Drawing for the job (mm, zero at the part's lowest x, y, z). Give positions to 0.01 mm unless a question says otherwise; leave off trailing zeros. Order: outer loops, then holes, each group sorted by start corner. A loop starts at its lowest first (then second) coordinate and runs counter-clockwise, first axis right, second up. Notation, with made-up numbers: (23, 77.5) -> (54, 77.5) arc R15 ccw to (54, 99.5) -> close; hole circle Ø8 at (36, -36). An arc over 180 degrees is marked (long way). One line per item, written item: value. Start each with the question number.
(1) Two-plate mould, pull along X, no slides. Class the marked faces 1, 2 and 3: +X half, -X half, draft (parallel to the pull), parting line (faces both ways), or undercut.
(2) Probe line 1 (Z direction, x = 21.5, y = 1.85); line 2 (Z direction, x = 17.5, y = 0.5); line 3 (Y direction, x = 17.5, z = 1.9). List the from-to ranges inside material, lowest first.
(3) Saw through at A-A on y = 2. Give the cut face in (x, z).
(4) Saw through at B-B on x = 16.75. Give the cut face in (y, z), plus the area to 3 significant figures.
(5) Pin check, flat tips, straight feed: pin 1 (0.6 mm diameter, centred on y = 1.5, z = 4, fed in from -X); pin 2 (1.5 mm diameter, centred on x = 14, z = 3, fed in from -Y); pin 3 (0.6 mm diameter, centred on y = 1.5, z = 3.5, fed in from +X); pin 4 (1 mm diameter, centred on x = 14, y = 1, fed in from -Z). Stop position of each tip, or through.
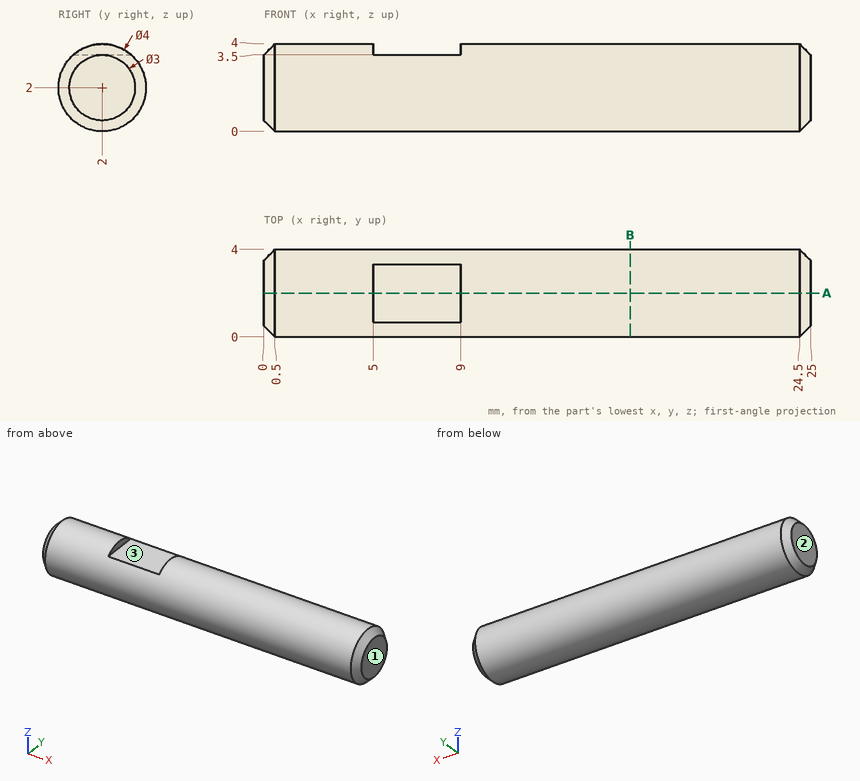
Results below:
1. face 1: +X half
1. face 2: -X half
1. face 3: undercut
2. line 1: z = 0.01 to 3.99
2. line 2: z = 0.68 to 3.32
2. line 3: y = 0 to 4
3. outline: (0, 0.5) -> (0.5, 0) -> (24.5, 0) -> (25, 0.5) -> (25, 3.5) -> (24.5, 4) -> (9, 4) -> (9, 3.5) -> (5, 3.5) -> (5, 4) -> (0.5, 4) -> (0, 3.5) -> close
4. outline: circle Ø4 at (2, 2)
4. area: 12.6 mm²
5. pin 1: stops at x = 0.26
5. pin 2: stops at y = 0.02
5. pin 3: stops at x = 25
5. pin 4: stops at z = 0.06
